from build123d import *

# Parameters (mm, degrees)
SKETCH_1_R          = 3.25
EXTRUDE_1_DEPTH     = 13
SKETCH_3_R          = 4.25
CUT_EXTRUDE_1_DEPTH = 17


with BuildPart() as part:
    # 草图1 → 凸台-拉伸1 (new, symmetric)
    with BuildSketch(Plane.XY):
        with BuildLine():
            Line((-77.585786438, 0), (0, 0))
            Line((0, 0), (0, 8))
            Line((0, 8), (-17.995464086, 8))
            Line((-17.995464086, 8), (-30.499317942, 38.186973559))
            Line((-30.499317942, 38.186973559), (-17.774603256, 50.911688245))
            Line((-17.774603256, 50.911688245), (-23.431457505, 56.568542495))
            Line((-23.431457505, 56.568542495), (-78.292893219, 1.707106781))
            ThreePointArc((-78.292893219, 1.707106781), (-78.50966597, 0.617316568), (-77.585786438, 0))
        make_face()
        with Locations(Location((-57.82689122, 9.184402377, 0), (0, 0, 180))):
            Circle(SKETCH_1_R, mode=Mode.SUBTRACT)
        Polygon((-67.928932188, 5), (-63.07447047, 5), (-64.496309389, 8.4326228), align=None, mode=Mode.SUBTRACT)
        with BuildLine():
            Line((-54.257468753, 5), (-20, 5))
            Line((-20, 5), (-34.038059223, 38.890872965))
            Line((-34.038059223, 38.890872965), (-58.261747684, 14.667184504))
            ThreePointArc((-58.261747684, 14.667184504), (-52.745553791, 11.289161255), (-54.257468753, 5))
        make_face(mode=Mode.SUBTRACT)
    extrude(amount=EXTRUDE_1_DEPTH, both=True)

    # 草图3 → 切除-拉伸1 (cut)
    with BuildSketch(Plane(origin=(0, 8, 0), x_dir=(1, 0, 0), z_dir=(0, 1, 0))):
        with Locations(Location((-10, 0, 0), (0, 0, 180))):
            Circle(SKETCH_3_R)
    cut_extrude_1 = extrude(amount=-CUT_EXTRUDE_1_DEPTH, mode=Mode.SUBTRACT)

    # 镜向1: 切除-拉伸1 across plane
    add(cut_extrude_1.mirror(Plane(origin=(-11.715728753, 28.284271247, 0), x_dir=(0, 0, 1), z_dir=(-0.3826834323650881, 0.9238795325112875, 0))), mode=Mode.SUBTRACT)


solid = part.part
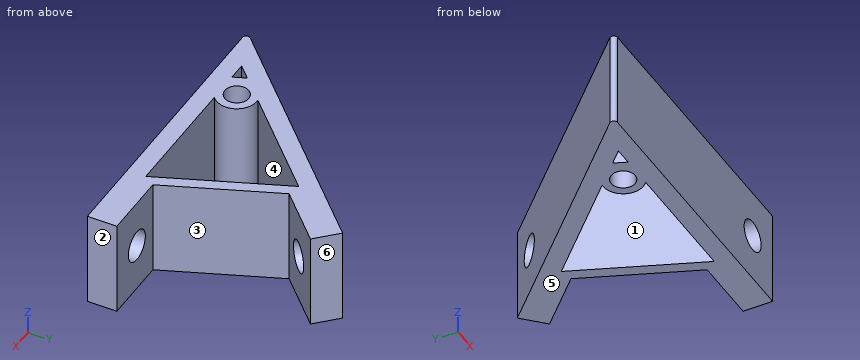
Verification items for the finished model (mm, model axes). Face numbers are marked on the shaded views. A direction names the side the tool comes from. Round coordinates to 2 decimals unless told otherwise and drop trailing zeros. Loops run counter-clockwise (first coordinate to the right, second up) from the corner with the lowest first, then second, coordinate; pieces in that order, holes last. Notation, with made-up numbers: M -37,55 L 11,55 A21 cw 11,63 Z; hole C 36.5,-6 d1. An arc over 180 degrees is marked long. Write each question's results on one line, items separated by ' | '.
1) Gauge pin test, flat ends, axial feed: P1, Ø8, axis at y = 46, z = -2.5, coming from the -X side; P2, Ø1.5, axis at y = 42, z = 5.5, coming from the -X side; P3, Ø9, axis at x = -10.5, z = -1.5, coming from the +Y side; P4, Ø6, axis at x = -57.83, y = 9.18, coming from the -Z side. Record the tip position at first contact, or that the pin passes through.
Checks:
P1: stops at x = -38 | P2: stops at x = -38.75 | P3: stops at y = 8 | P4: passes through
2) Access from +Z, -Z, +X, -X, +Y, -Y to the whole of each face (thin tool, end or side, straight path). Record for the marked faces 1, 2 and 3.
Checks:
face 1: +Z, -Z | face 2: +Z, -Z, +X, +Y, -Y | face 3: +Z, -Z, +X
3) Section check D-D on y = 34. Record the boundary of the cut face in (x, z).
Checks:
outline: M -46,-13 L -38.93,-13 L -38.93,13 L -46,13 Z; M -32.01,-13 L -28.77,-13 L -28.77,13 L -32.01,13 Z
4) Mould release check, pull along X, two halves, no side actions. Record for the marked faces 4, 5 and 6: released by +X, released by -X, zero draft, split by the parting line, or undercut.
Checks:
face 4: undercut | face 5: zero draft | face 6: released by +X
5) Section check C-C on y = 11. Record the boundary of the cut face in (x, z).
Checks:
outline: M -69,-13 L -60.52,-13 L -60.52,13 L -69,13 Z; M -55.13,-13 L -52.64,-13 L -52.64,13 L -55.13,13 Z; M -22.49,-13 L -19.24,-13 L -19.24,13 L -22.49,13 Z
6) Section check B-B on x = -10. Record the boundary of the cut face in (y, z), then the cut area to 3 significant figures.
Checks:
outline: M 0,-13 L 8,-13 L 8,-4.25 L 0,-4.25 Z; M 0,4.25 L 8,4.25 L 8,13 L 0,13 Z | area: 140 mm2
7) Section check A-A on z = 2.25. Record the boundary of the cut face in (x, y).
Checks:
outline: M -78.29,1.71 A1 ccw -77.59,0 L -13.61,0 L -13.61,8 L -18,8 L -30.5,38.19 L -27.4,41.29 L -33.05,46.95 Z; M -27.95,52.05 L -22.3,46.39 L -17.77,50.91 L -23.43,56.57 Z; M -6.39,0 L 0,0 L 0,8 L -6.39,8 Z; hole M -67.93,5 L -63.07,5 L -64.5,8.43 Z; hole C -57.83,9.18 d6.5; hole M -58.26,14.67 A5.5 cw -54.26,5 L -20,5 L -34.04,38.89 Z
8) Scan lines: L1, parallel to Z at x = -10, y = 2.5; L2, parallel to Y at x = -27, z = 3.5; L3, parallel to Y at x = -53, z = -9.5. Record each from-to range of solid material in increasing order. Write a range as from..to.
Checks:
L1: z = -13..-4.25, 4.25..13 | L2: y = 0..5, 21.9..29.74, 41.69..42.59, 49.4..53 | L3: y = 0..5, 6.55..11.82, 19.93..27
